from build123d import *

# Parameters (mm, degrees)
F2_SIZE2 = 0.25
F2_SIZE  = 0.25
F3_R     = 1
F5_DEPTH = 1.5


with BuildPart() as f1:
    # F0 (on Front) → F1 (revolve)
    with BuildSketch(Plane.XZ):
        Polygon((4.25, 0), (-4.25, 0), (-4.25, -1.65), (1.75, -1.65), (1.75, -3), (4.25, -3), align=None)
    revolve(axis=Axis((4.160319, 0, 0), (1, 0, 0)))

    # F2
    f2_edges = [f1.edges().sort_by_distance(p)[0] for p in [
        (-4.25, 0, 1.65),
    ]]
    chamfer(f2_edges, length=F2_SIZE, length2=F2_SIZE2)

    # F3
    f3_edges = [f1.edges().sort_by_distance(p)[0] for p in [
        (4.25, 0, 3),
    ]]
    fillet(f3_edges, radius=F3_R)

    # F4 (on face) → F5 (cut)
    with BuildSketch(Plane.YZ.offset(4.25)):
        Polygon((0.866025, 1.5), (-0.866025, 1.5), (-1.732051, 0), (-0.866025, -1.5), (0.866025, -1.5), (1.732051, 0), align=None)
    extrude(amount=-F5_DEPTH, mode=Mode.SUBTRACT)


solid = f1.part
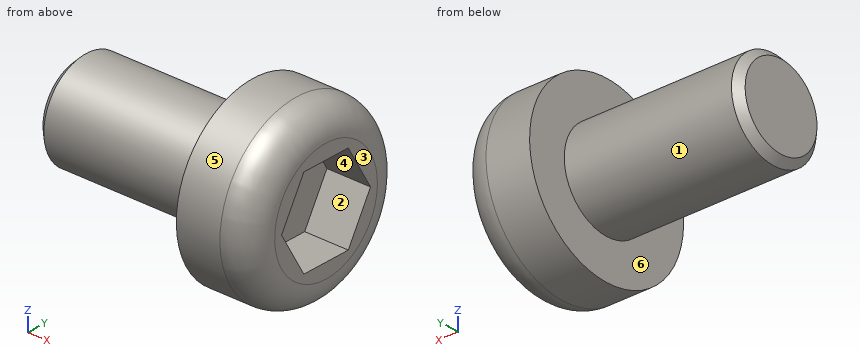
Verification items for the finished model (mm, model axes). Face numbers are marked on the shaded views. A direction names the side the tool comes from. Give positions to 0.01 mm unless a question says otherwise; leave off trailing zeros. Order: outer loops, then holes, each group sorted by start corner. A loop starts at its lowest first (then second) coordinate and runs counter-clockwise, first axis right, second up. Notation, with made-up numbers: M 6,12.5 L 12,12.5 A22 ccw 12,35.5 Z; hole C -38,23.25 d8. An arc over 180 degrees is marked long. Answer as a JSON object with one key per item and string values. Group by question number.
1) Cross-section at B-B (x = 0). Enter the section's corners in (y, z), then the cut area to 3 significant figures.
2) Scan lines: line 1 along X through (y, z) = (-1.75, -1); line 2 along X through (y, z) = (0.7, -0.5); line 3 along Z through (x, y) = (-2, 0.1). Record each from-to range of solid material in increasing order. Write a range as [from, to].
3) Mould release check, pull along Y, two halves, no side actions. Record for the marked faces 4, 5 and 6: released by +Y, released by -Y, zero draft, split by the parting line, or undercut.
4) Access from +Z, -Z, +X, -X, +Y, -Y to the whole of each face (thin tool, end or side, straight path). Record for the marked faces 1, 2 and 3.
5) Cross-section at A-A (y = 0). Enter the section's corners in (x, z), then the cut area to 3 significant figures.
6) Depth check by flat-ended pin: pin 1 Ø2 at (x, z) = (1, 1.5) entering from +Y; pin 2 Ø0.9 at (y, z) = (0.5, 0) entering from +X. Enter the tip coordinate at first touch or a pass-through.
Result sheet:
{
 "1": {"outline": "C 0,0 d3.3", "area": "8.55 mm2"},
 "2": {"line 1": "x = [1.75, 4.25]", "line 2": "x = [-4.25, 2.75]", "line 3": "z = [-1.65, 1.65]"},
 "3": {"face 4": "undercut", "face 5": "split by the parting line", "face 6": "zero draft"},
 "4": {"face 1": "-X", "face 2": "+X", "face 3": "+Z, -Z, +X, +Y, -Y"},
 "5": {"outline": "M -4.25,-1.4 L -4,-1.65 L 1.75,-1.65 L 1.75,-3 L 3.25,-3 A1 ccw 4.25,-2 L 4.25,-1.5 L 2.75,-1.5 L 2.75,1.5 L 4.25,1.5 L 4.25,2 A1 ccw 3.25,3 L 1.75,3 L 1.75,1.65 L -4,1.65 L -4.25,1.4 Z", "area": "29.8 mm2"},
 "6": {"pin 1": "stops at y = 2.88", "pin 2": "stops at x = 2.75"}
}
